```python
from build123d import *

# Parameters (mm, degrees)
SKETCH1_R           = 1.6
SKETCH1_R_2         = 11
SKETCH1_R_3         = 1.5
BOSS_EXTRUDE1_DEPTH = 3


with BuildPart() as part:
    # Sketch1 → Boss-Extrude1 (new body)
    with BuildSketch(Plane(origin=(0, 0, 0), x_dir=(1, 0, 0), z_dir=(0, 1, 0))):
        with BuildLine():
            Line((31.291637032, 13.44743291), (31.444863729, 13.535898385))
            ThreePointArc((31.444863729, 13.535898385), (32.908965344, 19), (27.444863729, 20.464101615))
            Line((27.444863729, 20.464101615), (27.291637032, 20.37563614))
            ThreePointArc((27.291637032, 20.37563614), (24.134706135, 19.749106847), (21.249974599, 21.176368422))
            ThreePointArc((21.249974599, 21.176368422), (0, 30), (-21.249974599, 21.176368422))
            ThreePointArc((-21.249974599, 21.176368422), (-24.134706135, 19.749106847), (-27.291637032, 20.37563614))
            Line((-27.291637032, 20.37563614), (-27.444863729, 20.464101615))
            ThreePointArc((-27.444863729, 20.464101615), (-32.92840763, 18.965940459), (-31.376555663, 13.49734868))
            ThreePointArc((-31.376555663, 13.49734868), (-29.189007561, 11.073540998), (-28.963860498, 7.816315311))
            ThreePointArc((-28.963860498, 7.816315311), (-25.980762114, -15), (-7.712802626, -28.991596639))
            ThreePointArc((-7.712802626, -28.991596639), (-5.004535966, -30.815192558), (-3.999230991, -33.921568627))
            ThreePointArc((-3.999230991, -33.921568627), (0, -38), (3.999230991, -33.921568627))
            ThreePointArc((3.999230991, -33.921568627), (5.004535966, -30.815192558), (7.712802626, -28.991596639))
            ThreePointArc((7.712802626, -28.991596639), (25.980378434, -15.000664533), (28.964260313, 7.814833621))
            ThreePointArc((28.964260313, 7.814833621), (29.170581299, 11.026715202), (31.291637032, 13.44743291))
        make_face()
        with Locations(Location((-29.444863729, 17, 0), (0, 0, 270))):
            Circle(SKETCH1_R, mode=Mode.SUBTRACT)
        with Locations(Location((29.444863729, 17, 0), (0, 0, 270))):
            Circle(SKETCH1_R, mode=Mode.SUBTRACT)
        with Locations(Location((0, -34, 0), (0, 0, 270))):
            Circle(SKETCH1_R, mode=Mode.SUBTRACT)
        with Locations(Location((0, 0, 0), (0, 0, 270))):
            Circle(SKETCH1_R_2, mode=Mode.SUBTRACT)
        with Locations(Location((-12.35, 7.130275824, 0), (0, 0, 270))):
            Circle(SKETCH1_R_3, mode=Mode.SUBTRACT)
        with Locations(Location((12.35, 7.130275824, 0), (0, 0, 270))):
            Circle(SKETCH1_R_3, mode=Mode.SUBTRACT)
        with Locations(Location((0, -14.260551649, 0), (0, 0, 270))):
            Circle(SKETCH1_R_3, mode=Mode.SUBTRACT)
    extrude(amount=BOSS_EXTRUDE1_DEPTH)


solid = part.part
```
Can you work these out from the model? Positions are in its coordinate system, mm. Give positions to 0.01 mm unless a question says otherwise; leave off trailing zeros. Loops run counter-clockwise (first coordinate to the right, second up) from the corner with the lowest first, then second, coordinate; pieces in that order, holes last. Notation, with made-up numbers: M -35,34 L -6,34 A33 ccw -6,69 Z; hole C -30,-0.75 d1. An arc over 180 degrees is marked long. One line per item, written item: value.
(1) Suppose I cut it at B-B on x = 0. List the corners of the cut face in (y, z) for me.
Returned:
outline: M 0,-30 L 3,-30 L 3,-11 L 0,-11 Z; M 0,11 L 3,11 L 3,12.76 L 0,12.76 Z; M 0,15.76 L 3,15.76 L 3,32.4 L 0,32.4 Z; M 0,35.6 L 3,35.6 L 3,38 L 0,38 Z
(2) Suppose I cut it at D-D on y = 1.45. List the corners of the cut face in (x, z) for me.
Returned:
outline: M -31.38,-13.5 A4 ccw long -27.44,-20.46 L -27.29,-20.38 A5 cw -21.25,-21.18 A30 ccw 21.25,-21.18 A5 cw 27.29,-20.38 L 27.44,-20.46 A4 ccw 31.44,-13.54 L 31.29,-13.45 A5 cw 28.96,-7.81 A30 ccw 7.71,28.99 A5 cw 4,33.92 A4 ccw long -4,33.92 A5 cw -7.71,28.99 A30 ccw -28.96,-7.82 A5 cw Z; hole C -29.44,-17 d3.2; hole C -12.35,-7.13 d3; hole C 0,0 d22; hole C 0,34 d3.2; hole C 0,14.26 d3; hole C 12.35,-7.13 d3; hole C 29.44,-17 d3.2
(3) Will this pin go through, and if not, where does the flat tip stop? pin 1 (1 mm diameter, centred on x = 8, y = 2.5, fed in from +Z).
Returned:
pin 1: z = 29.05
(4) I need wall thicknesses on line 1 (X direction, y = 2, z = -17); line 2 (X direction, y = 1.9, z = -17.5) (1 decimal); line 3 (Z direction, x = 7, y = 1.25). Which ranges of each line are inside material? Lowest first, please.
Returned:
line 1: -33.44 to -31.04, -27.84 to 27.84, 31.04 to 33.44
line 2: -33.4 to -31, -27.9 to 27.9, 31 to 33.4
line 3: -29.17 to -8.49, 8.49 to 29.24
(5) We'd pull the mould along X, two halves only. Please class faces 1 (the face through (-29.2, 1.5, -11.1)), 2 (the face through (-10.74, 1.48, -2.38)), 3 (the face through (28.47, 1.48, -18.27)), 4 (the face through (0, 3, -12)): released by +X, released by -X, zero draft, split by the parting line, or undercut.
Returned:
face 1: released by -X
face 2: undercut
face 3: undercut
face 4: zero draft
(6) Suppose I cut it at C-C on x = -12.35. List the corners of the cut face in (y, z) for me, plus the area to 3 significant figures.
Returned:
outline: M 0,-27.34 L 3,-27.34 L 3,-8.63 L 0,-8.63 Z; M 0,-5.63 L 3,-5.63 L 3,27.34 L 0,27.34 Z
area: 155 mm^2
(7) Suppose I cut it at A-A on z = 0. List the corners of the cut face in (x, y) for me, plus the area to 3 significant figures.
Returned:
outline: M -30,0 L -11,0 L -11,3 L -30,3 Z; M 11,0 L 30,0 L 30,3 L 11,3 Z
area: 114 mm^2
